```python
from build123d import *

# Parameters (mm, degrees)
SKETCH041_R              = 2.2
PAD010_DEPTH             = 20
SKETCH042_R              = 2.2
PAD011_DEPTH             = 20
SKETCH033_R              = 1.7
EXTRUDE002_DEPTH         = 10
SKETCH035_W              = 111
SKETCH035_H              = 60
PAD009_DEPTH             = 75
SKETCH036_W              = 73.889809
SKETCH036_H              = 62.1632
POCKET002008007007_DEPTH = 65
SKETCH037_W              = 53
SKETCH037_H              = 62.1458
POCKET002008007008_DEPTH = 10
SKETCH038_W              = 14.2
SKETCH038_H              = 53.6532
POCKET002008007009_DEPTH = 90
SKETCH039_W              = 45.91896
SKETCH039_H              = 44.45
POCKET002008007010_DEPTH = 15
SKETCH043_R              = 2.8
POCKET002008007011_DEPTH = 3.5
FILLET001008003_R        = 3


with BuildPart() as obj1:
    # Sketch041 → Pad010 (new body)
    with BuildSketch(Plane(origin=(82, 118.75, 168.7), x_dir=(0, 0, 1), z_dir=(1, 0, 0))):
        with Locations((-105.7463, 94.0605)):
            Circle(SKETCH041_R)
        with Locations((-105.7463, 83.9412)):
            Circle(SKETCH041_R)
        with Locations((-154.675, 83.9412)):
            Circle(SKETCH041_R)
        with Locations((-154.675, 94.0605)):
            Circle(SKETCH041_R)
        Polygon((-150.939961, 99.468416), (-109.632261, 99.468416), (-109.632261, 93), (-108, 92), (-108, 90.4953), (-105.472476, 90.4953), (-105.472476, 87.528957), (-108, 87.528957), (-108, 86), (-109.647222, 85), (-109.647222, 78.468416), (-150.954922, 78.468416), (-150.954922, 85), (-152.630008, 86.000023), (-152.630008, 87.528976), (-155.157516, 87.528976), (-155.157516, 90.45154), (-152.630008, 90.45154), (-152.630008, 92.000023), (-150.939961, 93), align=None)
    extrude(amount=PAD010_DEPTH)


with BuildPart() as obj2:
    # Sketch042 → Pad011 (new body)
    with BuildSketch(Plane(origin=(161.4, 118.75, 8), x_dir=(1, 0, 0), z_dir=(0, 0, -1))):
        with Locations((-105.7463, 94.0605)):
            Circle(SKETCH042_R)
        with Locations((-105.7463, 83.9412)):
            Circle(SKETCH042_R)
        with Locations((-154.675, 83.9412)):
            Circle(SKETCH042_R)
        with Locations((-154.675, 94.0605)):
            Circle(SKETCH042_R)
        Polygon((-150.939961, 99.468416), (-109.632261, 99.468416), (-109.632261, 93), (-108, 92), (-108, 90.4953), (-105.472476, 90.4953), (-105.472476, 87.528957), (-108, 87.528957), (-108, 86), (-109.647222, 85), (-109.647222, 78.468416), (-150.954922, 78.468416), (-150.954922, 85), (-152.630008, 86.000023), (-152.630008, 87.528976), (-155.157516, 87.528976), (-155.157516, 90.45154), (-152.630008, 90.45154), (-152.630008, 92.000023), (-150.939961, 93), align=None)
    extrude(amount=PAD011_DEPTH)


with BuildPart() as holes_servos_and_arduino:
    # Sketch033 → Extrude002 (new body)
    with BuildSketch(Plane.XY.offset(60)):
        with Locations((21.7411, 54.149063)):
            Circle(SKETCH033_R)
        with Locations((20.470995, 5.88126)):
            Circle(SKETCH033_R)
        with Locations((72.541618, 38.91581)):
            Circle(SKETCH033_R)
        with Locations((72.553482, 10.931391)):
            Circle(SKETCH033_R)
    extrude(amount=EXTRUDE002_DEPTH)


with BuildPart() as holes_servos_and_arduino_1:
    # Extrude002 placement: moved
    add(holes_servos_and_arduino.part.moved(Location((0, 0, 7))))

    # Fusion009003005002: union obj1, obj2
    add(obj1.part)
    add(obj2.part)


with BuildPart() as obj3:
    # Sketch035 → Pad009 (new body)
    with BuildSketch(Plane.XY):
        with Locations((55.5, 30)):
            Rectangle(SKETCH035_W, SKETCH035_H)
    extrude(amount=PAD009_DEPTH)

    # Sketch036 → Pocket002008007007 (cut)
    with BuildSketch(Plane.XZ):
        with Locations((46.039744, 37.56885)):
            Rectangle(SKETCH036_W, SKETCH036_H)
    extrude(amount=-POCKET002008007007_DEPTH, mode=Mode.SUBTRACT)

    # Sketch037 → Pocket002008007008 (cut)
    with BuildSketch(Plane(origin=(0, 0, 0), x_dir=(0, -1, 0), z_dir=(-1, 0, 0))):
        with Locations((-30, 37.56015)):
            Rectangle(SKETCH037_W, SKETCH037_H)
    extrude(amount=-POCKET002008007008_DEPTH, mode=Mode.SUBTRACT)

    # Sketch038 → Pocket002008007009 (cut)
    with BuildSketch(Plane.XY.offset(75)):
        with Locations((99.0507, 30)):
            Rectangle(SKETCH038_W, SKETCH038_H)
    extrude(amount=-POCKET002008007009_DEPTH, mode=Mode.SUBTRACT)

    # Sketch039 → Pocket002008007010 (cut)
    with BuildSketch(Plane.YZ.offset(111)):
        with Locations((30, 35.4627)):
            Rectangle(SKETCH039_W, SKETCH039_H)
    extrude(amount=-POCKET002008007010_DEPTH, mode=Mode.SUBTRACT)

    # Sketch043 → Pocket002008007011 (cut)
    with BuildSketch(Plane.YZ.offset(91.9507)):
        with Locations((24.666075, 62.980072)):
            Circle(SKETCH043_R)
        with Locations((34.802075, 62.980072)):
            Circle(SKETCH043_R)
        with Locations((24.666075, 13.932672)):
            Circle(SKETCH043_R)
        with Locations((34.745975, 13.932672)):
            Circle(SKETCH043_R)
    extrude(amount=-POCKET002008007011_DEPTH, mode=Mode.SUBTRACT)

    # Cut003: cut holes_servos_and_arduino
    add(holes_servos_and_arduino_1.part, mode=Mode.SUBTRACT)

    # Fillet001008003
    fillet001008003_edges = [obj3.edges().sort_by_distance(p)[0] for p in [
        (0, 0, 37.5),
        (55.5, 0, 0),
        (55.5, 0, 75),
        (111, 0, 37.5),
        (0, 60, 37.5),
        (0, 30, 0),
        (0, 30, 75),
        (111, 30, 0),
        (55.5, 60, 0),
        (111, 30, 75),
        (55.5, 60, 75),
        (111, 60, 37.5),
    ]]
    fillet(fillet001008003_edges, radius=FILLET001008003_R)


solid = obj3.part
```
The model under review builds one solid part; all positions refer to its coordinate system, in mm. A direction names the side the tool comes from. Round coordinates to 2 decimals unless told otherwise and drop trailing zeros. Order: outer loops, then holes, each group sorted by start corner. A loop starts at its lowest first (then second) coordinate and runs counter-clockwise, first axis right, second up.
Item 1: Add section B-B, the plane x = 104. State the section outline as (y, z) points.
Working result:
outline: (0, 3) arc R3 ccw to (3, 0) - (3.17, 0) - (3.17, 75) - (3, 75) arc R3 ccw to (0, 72) - close; (56.83, 0) - (57, 0) arc R3 ccw to (60, 3) - (60, 72) arc R3 ccw to (57, 75) - (56.83, 75) - close
Item 2: For pin 1 (1 mm diameter, centred on x = 19.5, y = 28, fed in from -Z); pin 2 (4 mm diameter, centred on y = 15, z = 39, fed in from -X); pin 3 (0.8 mm diameter, centred on y = 27.5, z = 2, fed in from +X), all flat-tipped, find the tip position at first contact; note any pin that passes through.
Working result:
pin 1: stops at z = 68.65
pin 2: stops at x = 82.98
pin 3: stops at x = 110.94
Item 3: Machinability: for faces 4 (the flat face through (46, 30, 68.65)), 5 (the flat face through (109, 30, 57.688)), 6 (the flat face through (87, 23, 17.76)), which of the approach directions +Z, -Z, +X, -X, +Y, -Y give a long, thin tool a straight path to every point of the face, cutting with its end or side? Answer none if there is none.
Working result:
face 4: +Y, -Y
face 5: +X
face 6: +X, -X
Item 4: To check wall thickness, follow probe 1 along X at (y, z) = (34.5, 4.5); probe 2 along Z at (x, y) = (86.5, 35); probe 3 along Y at (x, z) = (99, 29.5). State the ranges of each line that lie inside material, in increasing order.
Working result:
probe 1: x = 0 to 4.55, 8.9 to 10.45, 51.75 to 53.48, 57.83 to 91.95, 106.15 to 111
probe 2: z = 0 to 11.83, 16.22 to 17.75, 59.05 to 60.76, 65.15 to 75
probe 3: y = 0 to 3.17, 56.83 to 60
Item 5: Draft analysis for pull direction X (two halves, no side actions). For faces 1 (the flat face through (10.445, 37, 3)), 2 (the cylindrical face through (0.86, 0.9, 37.98)), 3 (the flat face through (55, 18, 0)), state which applies: released by +X, released by -X, zero draft, split by the parting line, or undercut.
Working result:
face 1: undercut
face 2: released by -X
face 3: zero draft
Item 6: Add section C-C, the plane y = 47. Count the separate pieces of the cut face and the enclosed holes in it, and give its area (3 significant figures).
Working result:
separate pieces: 3
enclosed holes: 0
area: 1,880 mm2
Item 7: Add section D-D, the plane x = 31. State the section outline as (y, z) points, and give its area (3 significant figures).
Working result:
outline: (0, 3) arc R3 ccw to (3, 0) - (19.28, 0) - (19.28, 6.49) - (0, 6.49) - close; (0, 68.65) - (60, 68.65) - (60, 72) arc R3 ccw to (57, 75) - (3, 75) arc R3 ccw to (0, 72) - close; (40.28, 0) - (57, 0) arc R3 ccw to (60, 3) - (60, 6.49) - (40.28, 6.49) - close
area: 626 mm2
Item 8: Add section A-A, the plane z = 9. State the section outline as (x, y) points, and give its area (3 significant figures).
Working result:
outline: (0, 3) arc R3 ccw to (3, 0) - (9.09, 0) - (9.09, 3.5) - (0, 3.5) - close; (0, 56.5) - (9.09, 56.5) - (9.09, 60) - (3, 60) arc R3 ccw to (0, 57) - close; (82.98, 0) - (108, 0) arc R3 ccw to (111, 3) - (111, 57) arc R3 ccw to (108, 60) - (82.98, 60) - close; hole (91.95, 3.17) - (106.15, 3.17) - (106.15, 56.83) - (91.95, 56.83) - close
area: 975 mm2
